Autodesk Inventor part; units mm, degrees
ref_plane "YZ Plane" through (0, 0, 0) normal (1, 0, 0) x (0, 1, 0)
ref_plane "XZ Plane" through (0, 0, 0) normal (0, 1, 0) x (-1, 0, 0)
ref_plane "XY Plane" through (0, 0, 0) normal (0, 0, 1) x (1, 0, 0)
sketch "Sketch1" plane through (0, 0, 0) normal (0, 1, 0) x (-1, 0, 0)
  circle A0 centre (0, 0) radius 32.5
  circle A1 centre (0, 0) radius 25
  circle A2 centre (17.3494, -18) radius 5
  circle A3 centre (18, 17.3494) radius 5
  circle A4 centre (-17.3494, 18) radius 5
  circle A5 centre (-18, -17.3494) radius 5
  line L0 (6, -18) -> (-6, -18) construction
  line L1 (6, -15.7639) -> (-6, -15.7639)
  line L2 (-6, -20.2361) -> (6, -20.2361)
  arc A6 (6, -20.2361) -> (6, -15.7639) centre (6, -18) ccw
  arc A7 (-6, -15.7639) -> (-6, -20.2361) centre (-6, -18) ccw
  line L3 (-25, 0) -> (25, 0) construction
  line L4 (6, 15.7639) -> (-6, 15.7639)
  line L5 (-6, 20.2361) -> (6, 20.2361)
  arc A8 (6, 15.7639) -> (6, 20.2361) centre (6, 18) ccw
  arc A9 (-6, 20.2361) -> (-6, 15.7639) centre (-6, 18) ccw
  circle A10 centre (0, 0) radius 37.5
  point P0 (0, -18)
  dimension "d0" = 65
  dimension "d1" = 50
  dimension "d2" = 10
  dimension "d5" = 360
  dimension "d7" = 35.3494
  dimension "d11" = 17.3494
  dimension "d12" = 11.3493
  dimension "d16" = 18
  dimension "d17" = 2.2361
  dimension "d18" = 18
  dimension "d19" = 75
extrude "Extrusion1" add sketch "Sketch1" against normal blind 10 contours A0 | A1 A2 A5 A4 A3
extrude "Extrusion2" add sketch "Sketch1" along normal blind 10 and the other way blind 10 contours A10
properties part number "case_top"
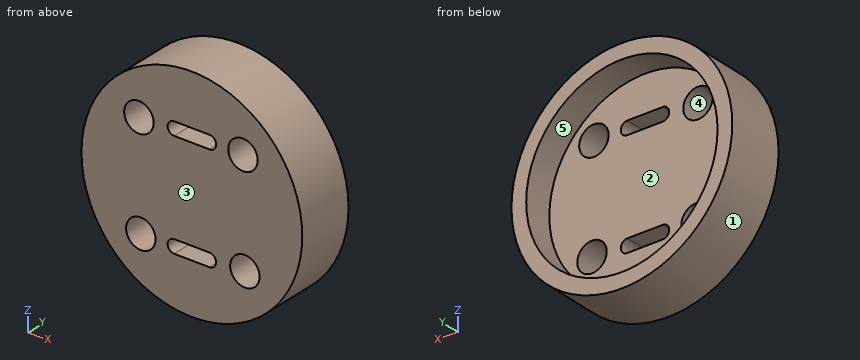
Design review of the part built by this model. Coordinates are the model's own, in mm. Face numbers are marked on the shaded views. A direction names the side the tool comes from. Coordinates: 2 decimals unless noted, no trailing zeros. Loops run counter-clockwise (first coordinate to the right, second up) from the corner with the lowest first, then second, coordinate; pieces in that order, holes last. Notation, with made-up numbers: (-21.5, 89) -> (-11.5, 89) arc R33 cw to (-11.5, 127) -> close; hole circle Ø11 at (51, 62). An arc over 180 degrees is marked (long way). Answer as a JSON object with one key per item and string values.
Q1. Clearance check with flat-ended pins moving along their axes: pin 1 Ø4 at (y, z) = (6, 28) entering from -X; pin 2 Ø5 at (x, y) = (-1.5, -7.5) entering from +Z; pin 3 Ø3 at (y, z) = (7.5, 5.5) entering from +X; pin 4 Ø12 at (y, z) = (1, 1) entering from +X. State where each tip first meets the part, or that it passes through.
Answer block:
{"pin 1": "stops at x = -27.02", "pin 2": "stops at z = 37.5", "pin 3": "stops at x = 37.29", "pin 4": "stops at x = 37.5"}
Q2. Tool access review of the marked faces 4 and 5: name each direction out of +Z, -Z, +X, -X, +Y, -Y from which nothing blocks a thin tool from reaching the whole face with its end or side.
Answer block:
{"face 4": "+Y, -Y", "face 5": "+Y"}
Q3. Take a section at D-D on z = 19. Give the boundary of the cut face in (x, y), plus the area to 3 significant figures.
Answer block:
{"outline": "(-32.33, -10) -> (-22.72, -10) -> (-22.72, 0) -> (-26.37, 0) -> (-26.37, 10) -> (-32.33, 10) -> close; (-13.28, -10) -> (-8, -10) -> (-8, 0) -> (-13.28, 0) -> close; (8, -10) -> (12.45, -10) -> (12.45, 0) -> (8, 0) -> close; (22.25, -10) -> (32.33, -10) -> (32.33, 10) -> (26.37, 10) -> (26.37, 0) -> (22.25, 0) -> close", "area": "413 mm^2"}
Q4. Take a section at B-B on z = 0. Give the boundary of the cut face in (x, y), plus the area to 3 significant figures.
Answer block:
{"outline": "(-37.5, -10) -> (37.5, -10) -> (37.5, 10) -> (32.5, 10) -> (32.5, 0) -> (-32.5, 0) -> (-32.5, 10) -> (-37.5, 10) -> close", "area": "850 mm^2"}
Q5. Take a section at C-C on y = 2.25. Give the boundary of the cut face in (x, z).
Answer block:
{"outline": "circle Ø75 at (0, 0); hole circle Ø65 at (0, 0)"}
Q6. Take a section at A-A on x = 0. Give the boundary of the cut face in (y, z), plus the area to 3 significant figures.
Answer block:
{"outline": "(-10, -37.5) -> (10, -37.5) -> (10, -32.5) -> (0, -32.5) -> (0, -20.24) -> (-10, -20.24) -> close; (-10, -15.76) -> (0, -15.76) -> (0, 15.76) -> (-10, 15.76) -> close; (-10, 20.24) -> (0, 20.24) -> (0, 32.5) -> (10, 32.5) -> (10, 37.5) -> (-10, 37.5) -> close", "area": "761 mm^2"}
Q7. The part is to be moulded in two halves that separate along X. For the marked faces 1, 2 and 3, say which applies: +X half, -X half, draft (parallel to the pull), parting line (faces both ways), or undercut.
Answer block:
{"face 1": "parting line", "face 2": "undercut", "face 3": "draft"}
Q8. To check wall thickness, follow L1, parallel to X at y = -6.25, z = -18; L2, parallel to Z at x = -18, y = -1.75; L3, parallel to X at y = -4, z = 18. State the ranges of each line that lie inside material, in increasing order.
Answer block:
{"L1": "x = -32.9 to -22.35, -12.35 to -8.24, 8.24 to 13.04, 22.96 to 32.9", "L2": "z = -32.9 to -22.96, -13.04 to 12.35, 22.35 to 32.9", "L3": "x = -32.9 to -22.96, -13.04 to -8.24, 8.24 to 12.35, 22.35 to 32.9"}
